The listing builds one solid part. Answer for the finished solid, in the listing's coordinates (mm). Face numbers are marked on the shaded views. A direction names the side the tool comes from. Give positions to 0.01 mm unless a question says otherwise; leave off trailing zeros. Order: outer loops, then holes, each group sorted by start corner. A loop starts at its lowest first (then second) coordinate and runs counter-clockwise, first axis right, second up. Notation, with made-up numbers: (33, 86) - (48, 86) arc R25 ccw to (48, 102) - close; hole circle Ø2 at (42, -30). An arc over 180 degrees is marked (long way). Use a Markdown table: item, result. Add a question column.
1) Find section D-D, the plane y = 43.5. Determine the outline of the cut face in (x, z), plus the area to 3 significant figures.
2) The mould has two halves that part along Z. Classify the marked faces 1, 2 and 3: released by +Z, released by -Z, zero draft, split by the parting line, or undercut.
3) For the marked faces 4, 5 and 6, determine the directions among +Z, -Z, +X, -X, +Y, -Y from which every point of the face is accessible in a straight line to the end or side of a thin tool.
4) Find section C-C, the plane x = 37. Determine the outline of the cut face in (y, z), plus the area to 3 significant figures.
5) Straight lines are drawn through the part: line 1 (X direction, y = 112.45, z = 0); line 2 (Y direction, x = 39.5, z = 10); line 3 (Y direction, x = -12.5, z = -6.5). For each, find the intervals that lie inside material, in ascending order.
6) Flat-ended cylindrical pins translate along their axes: pin 1 (10 mm diameter, centred on x = -23, z = 3.5, fed in from +Y); pin 2 (2 mm diameter, centred on y = 46.5, z = -2.5, fed in from +X); pin 3 (5 mm diameter, centred on x = 14.5, z = 16.5, fed in from -Y). Find the tip coordinate at first contact, or state that the pin passes through.
7) Find section B-B, the plane y = 107.5. Determine the outline of the cut face in (x, z).
from build123d import *

# Parameters (mm, degrees)
SKETCH1_R           = 5
BOSS_EXTRUDE1_DEPTH = 50
SKETCH2_R           = 10
BOSS_EXTRUDE2_DEPTH = 17.5
BOSS_EXTRUDE3_DEPTH = 7.5
SKETCH4_R           = 8.5
BOSS_EXTRUDE4_DEPTH = 16.5
SKETCH5_R           = 20
BOSS_EXTRUDE5_DEPTH = 10
SKETCH6_R           = 48.75
BOSS_EXTRUDE6_DEPTH = 12
CHAMFER1_SIZE2      = 10
CHAMFER1_SIZE       = 14.281480067
SKETCH7_R           = 43.75
CUT_EXTRUDE2_DEPTH  = 2
FILLET1_R           = 1


with BuildPart() as part:
    # Sketch1 → Boss-Extrude1 (new body)
    with BuildSketch(Plane(origin=(0, 0, 0), x_dir=(1, 0, 0), z_dir=(0, 1, 0))):
        with Locations(Location((0, 0, 0), (0, 0, 270))):
            Circle(SKETCH1_R)
    extrude(amount=BOSS_EXTRUDE1_DEPTH)

    # Sketch2 → Boss-Extrude2 (add)
    with BuildSketch(Plane(origin=(0, 50, 0), x_dir=(1, 0, 0), z_dir=(0, 1, 0))):
        with Locations(Location((0, 0, 0), (0, 0, 270))):
            Circle(SKETCH2_R)
    extrude(amount=BOSS_EXTRUDE2_DEPTH)

    # Sketch3 → Boss-Extrude3 (add)
    with BuildSketch(Plane(origin=(0, 67.5, 0), x_dir=(1, 0, 0), z_dir=(0, 1, 0))):
        Polygon((10.825317547, -6.25), (10.825317547, 6.25), (0, 12.5), (-10.825317547, 6.25), (-10.825317547, -6.25), (0, -12.5), align=None)
    extrude(amount=BOSS_EXTRUDE3_DEPTH)

    # Sketch4 → Boss-Extrude4 (add)
    with BuildSketch(Plane(origin=(0, 75, 0), x_dir=(1, 0, 0), z_dir=(0, 1, 0))):
        with Locations(Location((0, 0, 0), (0, 0, 270))):
            Circle(SKETCH4_R)
    extrude(amount=BOSS_EXTRUDE4_DEPTH)

    # Sketch5 → Boss-Extrude5 (add)
    with BuildSketch(Plane(origin=(0, 91.5, 0), x_dir=(1, 0, 0), z_dir=(0, 1, 0))):
        with Locations(Location((0, 0, 0), (0, 0, 270))):
            Circle(SKETCH5_R)
    extrude(amount=BOSS_EXTRUDE5_DEPTH)

    # Sketch6 → Boss-Extrude6 (add)
    with BuildSketch(Plane(origin=(0, 101.5, 0), x_dir=(1, 0, 0), z_dir=(0, 1, 0))):
        with Locations(Location((0, 0, 0), (0, 0, 270))):
            Circle(SKETCH6_R)
    extrude(amount=BOSS_EXTRUDE6_DEPTH)

    # Chamfer1
    chamfer1_edges = [part.edges().sort_by_distance(p)[0] for p in [
        (0, 101.5, -20),
    ]]
    chamfer1_side = [part.faces().sort_by_distance(p)[0] for p in [
        (0, 101.5, -20.2),
    ]]
    chamfer(chamfer1_edges, length=CHAMFER1_SIZE - 0.0001, length2=CHAMFER1_SIZE2 - 0.0001, reference=chamfer1_side[0])  # a hair under: the kernel refuses the full size

    # Sketch7 → Cut-Extrude2 (cut)
    with BuildSketch(Plane(origin=(0, 113.5, 0), x_dir=(1, 0, 0), z_dir=(0, 1, 0))):
        with Locations(Location((0, 0, 0), (0, 0, 270))):
            Circle(SKETCH7_R)
    extrude(amount=-CUT_EXTRUDE2_DEPTH, mode=Mode.SUBTRACT)

    # Fillet1
    fillet1_edges = [part.edges().sort_by_distance(p)[0] for p in [
        (0, 71.25, 12.5),
        (10.825317547, 71.25, 6.25),
        (10.825317547, 71.25, -6.25),
        (0, 71.25, -12.5),
        (-10.825317547, 71.25, -6.25),
        (-10.825317547, 71.25, 6.25),
        (0, 0, -5),
    ]]
    fillet(fillet1_edges, radius=FILLET1_R)


solid = part.part
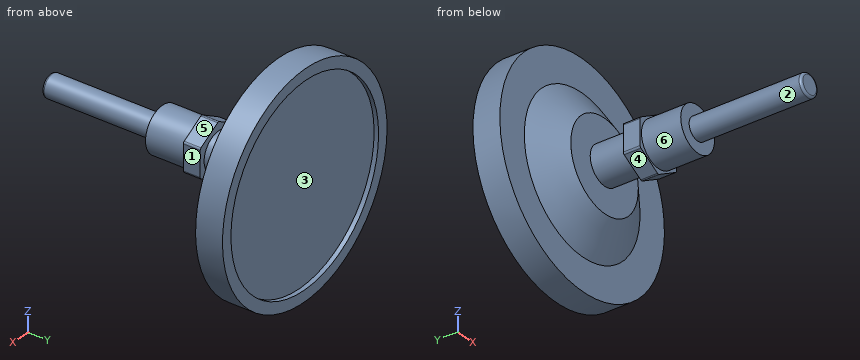
The answers:
| question | item | result |
|---|---|---|
| 1 | outline | circle Ø10 at (0, 0) |
| 1 | area | 78.5 mm2 |
| 2 | face 1 | zero draft |
| 2 | face 2 | split by the parting line |
| 2 | face 3 | undercut |
| 3 | face 4 | -Z, -X, -Y |
| 3 | face 5 | +Z, +X, -Y |
| 3 | face 6 | -Y |
| 4 | outline | (101.5, -31.74) - (113.5, -31.74) - (113.5, -23.35) - (111.5, -23.35) - (111.5, 23.35) - (113.5, 23.35) - (113.5, 31.74) - (101.5, 31.74) - close |
| 4 | area | 668 mm2 |
| 5 | line 1 | -48.75 to -43.75, 43.75 to 48.75 |
| 5 | line 2 | 101.5 to 111.5 |
| 5 | line 3 | 91.5 to 111.5 |
| 6 | pin 1 | y = 111.5 |
| 6 | pin 2 | x = 4.77 |
| 6 | pin 3 | y = 91.5 |
| 7 | outline | circle Ø97.5 at (0, 0) |
